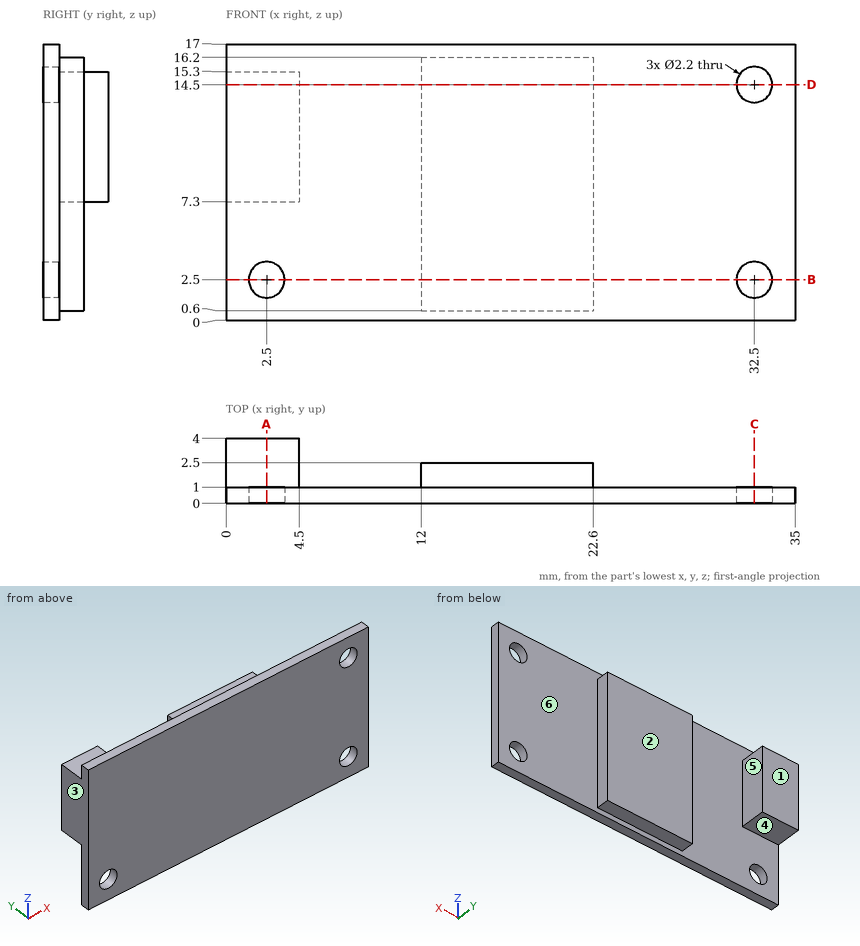
Geometry: see drawing. Coordinates: mm, zero at the bounding-box minimum. A direction names the side the tool comes from. Round coordinates to 2 decimals unless told otherwise and drop trailing zeros. Write each loop counter-clockwise with the first axis right and the second up, starting at its lowest first coordinate (ties: lowest second). Pieces come first, ordered by that corner, then holes.
1) Cut plane C-C (x = 32.5). Return the cut outline in (y, z).
2) Ray query, L1, parallel to Z at x = 32.5, y = 0.65; L2, parallel to X at y = 0.6, z = 2.5; L3, parallel to X at y = 0.2, z = 14.5. Return the intervals inside material, ascending.
3) Cut plane B-B (z = 2.5). Return the cut outline in (x, y).
4) Cut plane A-A (x = 2.5). Return the cut outline in (y, z), then the cut area to 3 significant figures.
5) Contact query for flat-ended pins moving along their axis: P1, Ø1.3, axis at x = 32.5, z = 2.5, coming from the -Y side; P2, Ø3, axis at x = 32.5, z = 14.5, coming from the +Y side; P3, Ø1.2, axis at x = 16.5, y = 2, coming from the -Z side; P4, Ø3, axis at x = 17.5, z = 9, coming from the +Y side. Output: stop coordinate, or through.
6) Draft query along X for the marked faces 3, 4, 5 and 6. Return one class per face: pulls with the +X half, pulls with the -X half, needs draft (parallel to the pull), parting line crosses it, or undercut.
7) Cut plane D-D (z = 14.5). Return the cut outline in (x, y), then the cut area to 3 significant figures.
8) Reachability of the marked faces 1 and 2 from +Z, -Z, +X, -X, +Y, -Y: full face, straight path, thin tool, end or side. Return the list, or none.
Geometry says:
1. outline: (0, 0) - (1, 0) - (1, 1.4) - (0, 1.4) - close; (0, 3.6) - (1, 3.6) - (1, 13.4) - (0, 13.4) - close; (0, 15.6) - (1, 15.6) - (1, 17) - (0, 17) - close
2. L1: z = 0 to 1.4, 3.6 to 13.4, 15.6 to 17
2. L2: x = 0 to 1.4, 3.6 to 31.4, 33.6 to 35
2. L3: x = 0 to 31.4, 33.6 to 35
3. outline: (0, 0) - (1.4, 0) - (1.4, 1) - (0, 1) - close; (3.6, 0) - (31.4, 0) - (31.4, 1) - (22.6, 1) - (22.6, 2.5) - (12, 2.5) - (12, 1) - (3.6, 1) - close; (33.6, 0) - (35, 0) - (35, 1) - (33.6, 1) - close
4. outline: (0, 0) - (1, 0) - (1, 1.4) - (0, 1.4) - close; (0, 3.6) - (1, 3.6) - (1, 7.3) - (4, 7.3) - (4, 15.3) - (1, 15.3) - (1, 17) - (0, 17) - close
4. area: 38.8 mm2
5. P1: passes through
5. P2: stops at y = 1
5. P3: stops at z = 0.6
5. P4: stops at y = 2.5
6. face 3: pulls with the -X half
6. face 4: needs draft
6. face 5: undercut
6. face 6: undercut
7. outline: (0, 0) - (31.4, 0) - (31.4, 1) - (22.6, 1) - (22.6, 2.5) - (12, 2.5) - (12, 1) - (4.5, 1) - (4.5, 4) - (0, 4) - close; (33.6, 0) - (35, 0) - (35, 1) - (33.6, 1) - close
7. area: 62.2 mm2
8. face 1: +Z, -Z, +X, -X, +Y
8. face 2: +Z, -Z, +X, +Y
